Read the model definition and answer for the solid it produces. Units are mm, in the model's axes. Coordinates: 2 decimals unless noted, no trailing zeros. Write each loop counter-clockwise with the first axis right and the second up, starting at its lowest first coordinate (ties: lowest second). Pieces come first, ordered by that corner, then holes.
from build123d import *

# Parameters (mm, degrees)
F0_R     = 8.89
F1_DEPTH = 25.4
F1_TAPER = 1
F2_T     = -0.508
F3_R     = 1.27


with BuildPart() as f1:
    # F0 (on Top) → F1 (new body)
    with BuildSketch(Plane.XY):
        Circle(F0_R)
    extrude(amount=F1_DEPTH, taper=F1_TAPER)

    # F2
    f2_openings = [f1.faces().sort_by_distance(p)[0] for p in [
        (0, 0, 0),
    ]]
    offset(amount=F2_T, openings=f2_openings)

    # F3
    f3_edges = [f1.edges().sort_by_distance(p)[0] for p in [
        (-8.446641, 0, 25.4),
    ]]
    fillet(f3_edges, radius=F3_R)


solid = f1.part
Item 1: Given pin 1 (5 mm diameter, centred on x = 3, y = -3, fed in from -Z); pin 2 (8 mm diameter, centred on x = -7, z = 6, fed in from -Y); pin 3 (2 mm diameter, centred on y = 6.5, z = 10.5, fed in from +X), each flat-ended and moving along its own axis, determine where each tip first touches the part or whether it passes through.
Item 2: Determine the mould class of faces 1 (the flat face through (0, 0, 24.892)), 2 (the flat face through (-3, 8, 0)), 3 (the conical face through (8.276, 2.606, 12.245)), 4 (the conical face through (4.39, 6.88, 12.62)) for opening direction X: +X half, -X half, draft (parallel to the pull), parting line (faces both ways), or undercut.
Item 3: The part is cut by section A-A (z = 12.75). Give the vertices of the cut face in (x, y).
Item 4: The part is cut by section B-B (z = 23). Give the vertices of the cut face in (x, y), and give its area (3 significant figures).
Item 5: Find the intervals of material crossed by probe 1 along Z at (x, y) = (1.5, 4.5); probe 2 along X at (y, z) = (-2.25, 18.25); probe 3 along X at (y, z) = (-2.25, 2.25), in increasing order.
Answer:
1. pin 1: stops at z = 24.89
1. pin 2: stops at y = -8.26
1. pin 3: stops at x = 6.75
2. face 1: undercut
2. face 2: draft
2. face 3: parting line
2. face 4: undercut
3. outline: circle Ø17.33 at (0, 0); hole circle Ø16.32 at (0, 0)
4. outline: circle Ø16.98 at (0, 0); hole circle Ø15.96 at (0, 0)
4. area: 26.3 mm2
5. probe 1: z = 24.89 to 25.4
5. probe 2: x = -8.27 to -7.74, 7.74 to 8.27
5. probe 3: x = -8.56 to -8.03, 8.03 to 8.56
